```python
from build123d import *

# Parameters (mm, degrees)
F0_R     = 10
F1_DEPTH = 25
F2_DEPTH = 50
F3_SIZE  = 2
F4_R     = 40.723122
F5_DEPTH = 50.493211


with BuildPart() as f1:
    # F0 (on Front) → F1 (new body)
    with BuildSketch(Plane.XZ):
        with BuildLine():
            ThreePointArc((2.083333, -24.913043), (18.399502, -16.92508), (25, 0))
            ThreePointArc((25, 0), (18.399502, 16.92508), (2.083333, 24.913043))
            ThreePointArc((2.083333, 24.913043), (-25, 0), (2.083333, -24.913043))
        make_face()
        Circle(F0_R, mode=Mode.SUBTRACT)
        with BuildLine():
            ThreePointArc((2.083333, 24.913043), (18.399502, 16.92508), (25, 0))
            ThreePointArc((25, 0), (18.399502, -16.92508), (2.083333, -24.913043))
            Line((2.083333, -24.913043), (91.458333, -17.43913))
            ThreePointArc((91.458333, -17.43913), (72.5, 0), (91.458333, 17.43913))
            Line((91.458333, 17.43913), (2.083333, 24.913043))
        make_face()
        with BuildLine():
            ThreePointArc((107.5, 0), (102.879651, 11.847556), (91.458333, 17.43913))
            ThreePointArc((91.458333, 17.43913), (72.5, 0), (91.458333, -17.43913))
            ThreePointArc((91.458333, -17.43913), (102.879651, -11.847556), (107.5, 0))
        make_face()
        with Locations((90, 0)):
            Circle(F0_R, mode=Mode.SUBTRACT)
    extrude(amount=F1_DEPTH)

    # F0 (on Front) → F2 (join)
    with BuildSketch(Plane.XZ):
        with BuildLine():
            ThreePointArc((2.083333, -24.913043), (18.399502, -16.92508), (25, 0))
            ThreePointArc((25, 0), (18.399502, 16.92508), (2.083333, 24.913043))
            ThreePointArc((2.083333, 24.913043), (-25, 0), (2.083333, -24.913043))
        make_face()
        Circle(F0_R, mode=Mode.SUBTRACT)
    extrude(amount=F2_DEPTH)

    # F3
    f3_edges = [f1.edges().sort_by_distance(p)[0] for p in [
        (-2.083333, -50, 24.913043),
        (-10, -50, 0),
        (80, -25, 0),
    ]]
    chamfer(f3_edges, length=F3_SIZE)

    # F4 (on Front) → F5 (join)
    with BuildSketch(Plane.XZ):
        Circle(F4_R)
    extrude(amount=-F5_DEPTH)


solid = f1.part
```
Check sheet for the modelled part. Datum: model origin and axes. Units: mm. A direction names the side the tool comes from. Round coordinates to 2 decimals unless told otherwise and drop trailing zeros. Order: outer loops, then holes, each group sorted by start corner. A loop starts at its lowest first (then second) coordinate and runs counter-clockwise, first axis right, second up.
1) Go/stop test with flat-tipped pins: pin 1 Ø12 at (y, z) = (-38.5, -3) entering from +X; pin 2 Ø16 at (x, z) = (2.5, 3) entering from -Y; pin 3 Ø8 at (y, z) = (10, 29) entering from -X. Record where each tip stops, or that it passes through.
2) Section check C-C (y = 20). Record the boundary of the cut face in (x, z).
3) Section check A-A (y = -18). Record the boundary of the cut face in (x, z), and give its area (3 significant figures).
4) Mould release check, pull along Z, two halves, no side actions. Record for faces 5 (the flat face through (10, -50, -10)), 6 (the cylindrical face through (80, -11, 0)), 7 (the flat face through (47.396, -12.325, 21.124)): +Z half, -Z half, draft (parallel to the pull), parting line (faces both ways), or undercut.
5) Scan lines: line 1 (Z direction, x = 0, y = -35); line 2 (Y direction, x = 16, z = -30.5); line 3 (Y direction, x = 25.5, z = -22.5). Record each from-to range of solid material in increasing order.
6) Section check B-B (x = 0). Record the boundary of the cut face in (y, z).
7) Tool access check on faces 1 (the flat face through (-1, 50.493, 1)), 2 (the flat face through (46.15, -12.32, -21.23)), 3 (the cylindrical face through (-2.17, -23.66, -9.76)), 4 (the cylindrical face through (-5.301, 24.893, 40.377)). Record the directions out of +Z, -Z, +X, -X, +Y, -Y that give a thin tool (end or side, any length) a straight path to the whole face; none if there is none.
8) Section check D-D (z = 34.5). Record the boundary of the cut face in (x, y), and give its area (3 significant figures).
Result:
1. pin 1: stops at x = 25
1. pin 2: stops at y = -49.91
1. pin 3: stops at x = -32.15
2. outline: circle Ø81.45 at (0, 0)
3. outline: (2.08, -24.91) - (91.46, -17.44) arc R17.5 ccw to (91.46, 17.44) - (2.08, 24.91) arc R25 ccw (long way) to start; hole circle Ø20 at (0, 0); hole circle Ø20 at (90, 0)
3. area: 4,670 mm2
4. face 5: draft
4. face 6: undercut
4. face 7: +Z half
5. line 1: z = -25 to -10, 10 to 25
5. line 2: y = 0 to 50.49
5. line 3: y = -25 to 50.49
6. outline: (-50, -23) - (-48, -25) - (0, -25) - (0, -40.72) - (50.49, -40.72) - (50.49, 40.72) - (0, 40.72) - (0, 25) - (-48, 25) - (-50, 23) - (-50, 12) - (-48, 10) - (0, 10) - (0, -10) - (-48, -10) - (-50, -12) - close
7. face 1: +Z, -Z, +X, -X, +Y
7. face 2: -Z, +X, -Y
7. face 3: -Y
7. face 4: +Y
8. outline: (-21.64, 0) - (21.64, 0) - (21.64, 50.49) - (-21.64, 50.49) - close
8. area: 2,180 mm2
